Geometry check sheet. Reference: the model listing, model coordinates, mm. Face numbers are marked on the shaded views. A direction names the side the tool comes from. Round coordinates to 2 decimals unless told otherwise and drop trailing zeros. Loops run counter-clockwise (first coordinate to the right, second up) from the corner with the lowest first, then second, coordinate; pieces in that order, holes last. Notation, with made-up numbers: (37, -31) - (49, -31) arc R24 cw to (49, -12) - close; hole circle Ø9 at (37.25, -7). An arc over 180 degrees is marked (long way). Answer in a Markdown table with one row per item. Add a question column.
```python
from build123d import *

# Parameters (mm, degrees)
SKETCH2_R          = 4
CUT_EXTRUDE1_DEPTH = 12
CUT_EXTRUDE2_REACH = 74
SKETCH3_R          = 4


with BuildPart() as part:
    # Sketch1 → Revolve1 (revolve)
    with BuildSketch(Plane.XY):
        Polygon((-25.700460829, 11.1), (-25.700460829, 24), (-1.700460829, 24), (-1.700460829, 48), (10.299539171, 48), (10.299539171, 11.1), align=None)
    revolve(axis=Axis((-11.612903226, 0, 0), (1, 0, 0)))

    # Sketch2 → Cut-Extrude1 (cut)
    with BuildSketch(Plane.ZY.offset(1.700460829)):
        with Locations((0, 36)):
            Circle(SKETCH2_R)
        with Locations((31.176914536, 18)):
            Circle(SKETCH2_R)
        with Locations((31.176914536, -18)):
            Circle(SKETCH2_R)
        with Locations((0, -36)):
            Circle(SKETCH2_R)
        with Locations((-31.176914536, -18)):
            Circle(SKETCH2_R)
        with Locations((-31.176914536, 18)):
            Circle(SKETCH2_R)
    extrude(amount=-CUT_EXTRUDE1_DEPTH, mode=Mode.SUBTRACT)

    # Sketch3 → Cut-Extrude2 (cut, up to next)
    with BuildSketch(Plane.XY.offset(24), mode=Mode.PRIVATE) as cut_extrude2_sk1:
        with Locations((-13.700460829, 0)):
            Circle(SKETCH3_R)
    cut_extrude2_tool1 = extrude(cut_extrude2_sk1.sketch, amount=-CUT_EXTRUDE2_REACH, mode=Mode.PRIVATE) & part.part
    add(cut_extrude2_tool1.solids().sort_by_distance((-13.700461, 0, 24))[0], mode=Mode.SUBTRACT)


solid = part.part
```
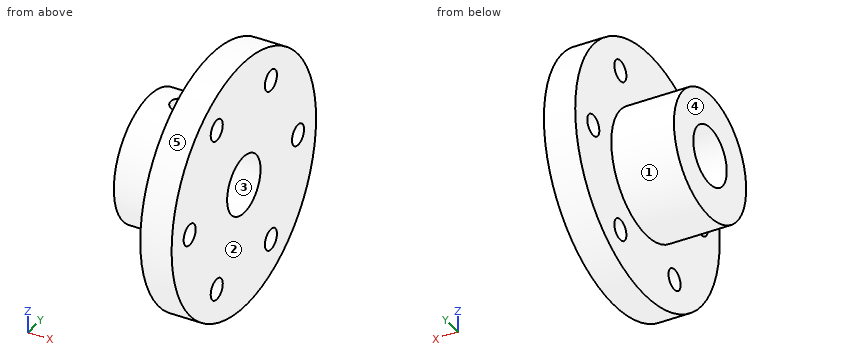
Q1. Cross-section at A-A, the plane y = 0. Enter the section's corners in (x, z), plus the area to 3 significant figures.
Q2. Cross-section at B-B, the plane z = 0. Enter the section's corners in (x, y), plus the area to 3 significant figures.
Q3. Set-up check for the marked faces 1 and 2: record each of +Z, -Z, +X, -X, +Y, -Y from which the full face is reachable in a straight line by a thin tool's end or side.
Q4. Release check for a two-part mould opening along Z. For the marked faces 3, 4 and 5 record: +Z half, -Z half, draft (parallel to the pull), parting line (faces both ways), or undercut.
Q5. Depth check by flat-ended pin: P1, Ø1.5, axis at x = 2, y = 16.5, coming from the -Z side; P2, Ø7, axis at y = -36, z = 0, coming from the -X side; P3, Ø9, axis at y = -18, z = 31.18, coming from the -X side; P4, Ø10.5, axis at x = -13.7, y = 0, coming from the +Z side. Enter the tip coordinate at first touch or a pass-through.
Q6. Cross-section at C-C, the plane y = -36. Enter the section's corners in (x, z), plus the area to 3 significant figures.
Q7. Cross-section at D-D, the plane x = -3. Enter the section's corners in (y, z), plus the area to 3 significant figures.
Q8. Scan lines: line 1 (X direction, y = 33, z = -29); line 2 (Z direction, x = 3.5, y = 16.5); line 3 (Z direction, x = -18, y = 0). Record each from-to range of solid material in increasing order. Write a range as from..to.
Check sheet entries:
| question | item | result |
|---|---|---|
| 1 | outline | (-25.7, -24) - (-1.7, -24) - (-1.7, -48) - (10.3, -48) - (10.3, -11.1) - (-25.7, -11.1) - close; (-25.7, 11.1) - (-17.7, 11.1) - (-17.7, 24) - (-25.7, 24) - close; (-9.7, 11.1) - (10.3, 11.1) - (10.3, 48) - (-1.7, 48) - (-1.7, 24) - (-9.7, 24) - close |
| 1 | area | 1,400 mm² |
| 2 | outline | (-25.7, -24) - (-1.7, -24) - (-1.7, -32) - (10.3, -32) - (10.3, -11.1) - (-25.7, -11.1) - close; (-25.7, 11.1) - (10.3, 11.1) - (10.3, 32) - (-1.7, 32) - (-1.7, 24) - (-25.7, 24) - close; (-1.7, -48) - (10.3, -48) - (10.3, -40) - (-1.7, -40) - close; (-1.7, 40) - (10.3, 40) - (10.3, 48) - (-1.7, 48) - close |
| 2 | area | 1,310 mm² |
| 3 | face 1 | -X |
| 3 | face 2 | +Z, -Z, +X, +Y, -Y |
| 4 | face 3 | undercut |
| 4 | face 4 | draft |
| 4 | face 5 | parting line |
| 5 | P1 | z = -45.34 |
| 5 | P2 | through |
| 5 | P3 | x = -1.7 |
| 5 | P4 | z = 24 |
| 6 | outline | (-1.7, -31.75) - (10.3, -31.75) - (10.3, -4) - (-1.7, -4) - close; (-1.7, 4) - (10.3, 4) - (10.3, 31.75) - (-1.7, 31.75) - close |
| 6 | area | 666 mm² |
| 7 | outline | circle Ø48 at (0, 0); hole circle Ø22.2 at (0, 0) |
| 7 | area | 1,420 mm² |
| 8 | line 1 | -1.7..10.3 |
| 8 | line 2 | -45.07..-34.89, -27.47..27.47, 34.89..45.07 |
| 8 | line 3 | -24..-11.1, 11.1..24 |
